For this review, take the finished solid that the model builds, in its own axes (mm). Round coordinates to 2 decimals unless told otherwise and drop trailing zeros. Write each loop counter-clockwise with the first axis right and the second up, starting at its lowest first coordinate (ties: lowest second). Pieces come first, ordered by that corner, then holes. Notation, with made-up numbers: (46.25, 44.5) -> (94.25, 44.5) arc R22 cw to (94.25, 72.5) -> close; hole circle Ø8 at (40, 10.25). An arc over 180 degrees is marked (long way). Answer as CSV lines item,"result". Start each with the question number.
Item 1: Take a section at C-C on y = -1.7. Give the boundary of the cut face in (x, z).
Item 2: Wall thickness on probe 1 along Z at (x, y) = (2.25, -0.6); probe 2 along Z at (x, y) = (-8, -1.6); probe 3 along X at (y, z) = (-1, -0.5): over which ranges is each line inside the solid? List them lowest first. Write a range as from..to.
Item 3: Take a section at B-B on x = 0. Give the boundary of the cut face in (y, z).
Item 4: Take a section at D-D on z = 12.5. Give the boundary of the cut face in (x, y), then the cut area to 3 significant figures.
Item 5: Take a section at A-A on z = 0. Give the boundary of the cut face in (x, y).
Item 6: For pin 1 Ø1 at (y, z) = (-0.5, 1) entering from -X, flat-tipped, find the tip position at first contact; note if it passes through.
Solid Edge part; units mm, degrees
sketch "Sketch1" plane through (0, 0, 0) normal (0, -1, 0) x (1, 0, 0)
  arc A0 (-6.0052, 8.3067) -> (-10.25, 21.4237) centre (-10.25, 14.1784) ccw
  arc A1 (-10.25, 21.4237) -> (10.25, 21.4237) centre (0, 4.25) cw
  arc A2 (10.25, 21.4237) -> (6.0052, 8.3067) centre (10.25, 14.1784) ccw
  arc A3 (6.0052, 8.3067) -> (-6.0052, 8.3067) centre (0, 0) cw
  dimension "D1" = 6.0052
extrude "Protrusion1" add sketch "Sketch1" along normal blind 2
sketch "Sketch2" plane through (0, -2, 7) normal (0, -1, 0) x (1, 0, 0)
  line L0 (-4, -3) -> (4, -3)
  line L1 (4, -3) -> (4, -11)
  line L2 (4, -11) -> (-4, -11)
  line L3 (-4, -11) -> (-4, -3)
  dimension "D1" = 4
  dimension "D2" = 4
extrude "Cutout1" cut sketch "Sketch2" against normal through all
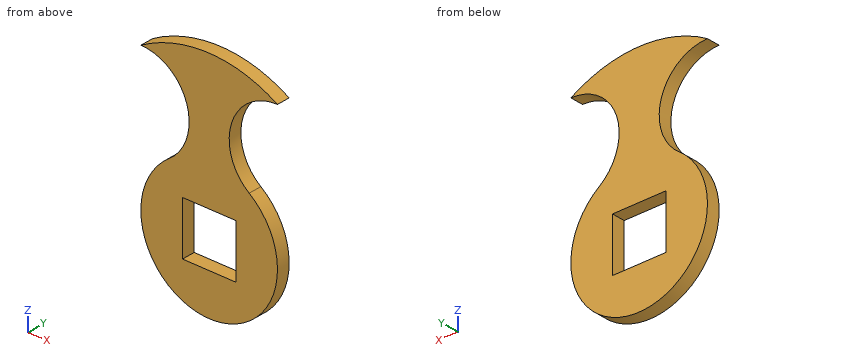
Output values:
1,outline,"(-10.25, 21.42) arc R7.25 cw to (-6.01, 8.31) arc R10.25 ccw (long way) to (6.01, 8.31) arc R7.25 cw to (10.25, 21.42) arc R20 ccw to start; hole (-4, -4) -> (4, -4) -> (4, 4) -> (-4, 4) -> close"
2,probe 1,"z = -10..-4, 4..24.12"
2,probe 2,"z = -6.41..6.41, 21.07..22.58"
2,probe 3,"x = -10.24..-4, 4..10.24"
3,outline,"(-2, -10.25) -> (0, -10.25) -> (0, -4) -> (-2, -4) -> close; (-2, 4) -> (0, 4) -> (0, 24.25) -> (-2, 24.25) -> close"
4,outline,"(-3.2, -2) -> (3.2, -2) -> (3.2, 0) -> (-3.2, 0) -> close"
4,area,"12.8 mm^2"
5,outline,"(-10.25, -2) -> (-4, -2) -> (-4, 0) -> (-10.25, 0) -> close; (4, -2) -> (10.25, -2) -> (10.25, 0) -> (4, 0) -> close"
6,pin 1,"stops at x = -10.24"
